Autodesk Inventor part; units mm, degrees
ref_plane "Work Plane1" through (4.4177, 0, 646.75) normal (0, 1, 0) x (1, 0, 0)
ref_plane "YZ Plane" through (0, 0, 0) normal (1, 0, 0) x (0, 1, 0)
ref_plane "XZ Plane" through (0, 0, 0) normal (0, 1, 0) x (-1, 0, 0)
sketch "Sketch1" plane through (0, 0, 0) normal (0, 0, 1) x (1, 0, 0)
  line L0 (4.4177, -4.0601) -> (-4.4177, -4.0601)
  line L1 (-4.4177, -4.0601) -> (-4.4177, 4.0601)
  line L2 (-4.4177, 4.0601) -> (4.4177, 4.0601)
  line L3 (4.4177, 4.0601) -> (4.4177, -4.0601)
  line L4 (4.4177, -4.0601) -> (-4.4177, 4.0601) construction
  line L5 (-4.4177, -4.0601) -> (4.4177, 4.0601) construction
  point P0 (0, 0)
extrude "Extrusion1" add sketch "Sketch1" along normal blind 650
fillet "Fillet2" radius 3.25 4 edges at (0, 4.0601, 650) (-4.4177, 0, 650) (0, -4.0601, 650) (4.4177, 0, 650)
ref_plane "Work Plane1" through (4.4177, 0, 646.75) normal (0, 1, 0) x (1, 0, 0)
sketch "Sketch2" plane through (4.4177, 0, 646.75) normal (0, 1, 0) x (1, 0, 0)
  line L0 (-8.8354, 0) -> (0, 0)
  arc A0 (-8.8354, 0) -> (0, 0) centre (-4.4177, 1.3775) ccw
  line L1 (-8.8354, 0) -> (-8.8354, -4.2008)
  line L2 (-8.8354, -4.2008) -> (-4.4177, -4.2008)
  line L3 (-4.4177, -4.2008) -> (-4.4177, -3.25)
  point P0 (-4.4177, 646.75)
extrude "Extrusion2" cut sketch "Sketch2" along normal mid plane 20 contours L0 A0
sketch "Sketch3" plane through (4.4177, 4.0601, 646.75) normal (0, 1, 0) x (1, 0, 0)
  line L0 (-9.2871, 0) -> (1.4537, 0)
  line L1 (1.4537, 0) -> (1.4537, -3.6122)
  line L2 (1.4537, -3.6122) -> (-9.2871, -3.6122)
  line L3 (-9.2871, -3.6122) -> (-9.2871, 0)
  point P0 (-4.4177, 646.75)
extrude "Extrusion3" cut sketch "Sketch3" against normal blind 25.5
sketch "Sketch4" plane through (4.4177, 4.0601, 646.75) normal (0, 1, 0) x (1, 0, 0)
  line L0 (-8.8354, 0) -> (0, 0)
  arc A0 (-8.8354, 0) -> (0, 0) centre (-4.4177, 0.2318) ccw
  point P0 (-4.4177, 646.75)
extrude "Extrusion4" add sketch "Sketch4" against normal blind 8.25
sketch "Sketch5" plane through (0, 0, 0) normal (0, 0, -1) x (-1, 0, 0)
  line L0 (-450, 35) -> (450, 35)
  line L1 (450, 35) -> (450, -35)
  line L2 (450, -35) -> (-450, -35)
  line L3 (-450, -35) -> (-450, 35)
  line L4 (-450, 35) -> (450, -35) construction
  line L5 (450, 35) -> (-450, -35) construction
  circle A0 centre (161.6649, 0) radius 5
  circle A1 centre (-379.6072, 0) radius 5
  point P0 (0, 0)
  dimension "d11" = 900
  dimension "d12" = 70
  dimension "d14" = 10
extrude "Extrusion5" add sketch "Sketch5" along normal blind 10
extrude "Extrusion6" add sketch "Sketch5" along normal blind 658.25 contours A0 | A1
Design review of the part built by this model. Coordinates are the model's own, in mm. Round coordinates to 2 decimals unless told otherwise and drop trailing zeros. Loops run counter-clockwise (first coordinate to the right, second up) from the corner with the lowest first, then second, coordinate; pieces in that order, holes last. Notation, with made-up numbers: (86.5, 75) -> (129.5, 75) arc R26 cw to (129.5, 111) -> close; hole circle Ø3 at (66.25, 84). An arc over 180 degrees is marked (long way). Use one line per item in the form item = value. Start each with the question number.
Q1. We need section C-C on y = 18. Give the boundary of the cut face in (x, z).
Q2. We need section B-B on z = 402.5. Give the boundary of the cut face in (x, y).
Q3. Wall thickness on line 1 along Z through (x, y) = (116, 16.5): over which ranges is the line inside the solid? List them lowest first. Write a range as [from, to].
Q4. We need section A-A on z = -29. Give the boundary of the cut face in (x, y).
Q5. For pin 1 Ø1 at (x, y) = (-199, -6) entering from +Z; pin 2 Ø3 at (y, z) = (-1, -329) entering from -X; pin 3 Ø2.5 at (y, z) = (-1, 392) entering from +X, all flat-tipped, find the tip position at first contact; note any pin that passes through.
Calculated:
q1.outline = (-450, -10) -> (450, -10) -> (450, 0) -> (-450, 0) -> close
q2.outline = (-4.42, -4.06) -> (4.42, -4.06) -> (4.42, 4.06) -> (-4.42, 4.06) -> close
q3.line_1 = [-10, 0]
q4.outline = circle Ø10 at (-161.66, 0); circle Ø10 at (379.61, 0)
q5.pin_1 = 0
q5.pin_2 = -166.66
q5.pin_3 = 4.42
